Check sheet for the drawn part. Datum: minimum x, y, z corner. Units: mm. Round coordinates to 2 decimals unless told otherwise and drop trailing zeros. Write each loop counter-clockwise with the first axis right and the second up, starting at its lowest first coordinate (ties: lowest second). Pieces come first, ordered by that corner, then holes. Notation, with made-up numbers: (6.5, 12) - (64.5, 12) arc R8 cw to (64.5, 20) - close; hole circle Ø7 at (68.25, 68). An arc over 180 degrees is marked (long way). Answer as a JSON object with one key per item and string values. Group by question number.
Item 1: Sectioned sample at C-C on y = 1.1. Record the boundary of the cut face in (x, z), plus the area to 3 significant figures.
Item 2: Sectioned sample at B-B on z = 8. Record the boundary of the cut face in (x, y), plus the area to 3 significant figures.
Item 3: Sectioned sample at A-A on x = 8. Record the boundary of the cut face in (y, z).
Item 4: Release check for a two-part mould opening along Z. For the marked faces 1, 2, 3 and 4 record: pulls with the +Z half, pulls with the -Z half, needs draft (parallel to the pull), parting line crosses it, or undercut.
Item 5: Thickness scan on line 1 (X direction, y = 0.4, z = 8); line 2 (Z direction, x = 6.5, y = 1.25). Record the ranges inside material, lowest first.
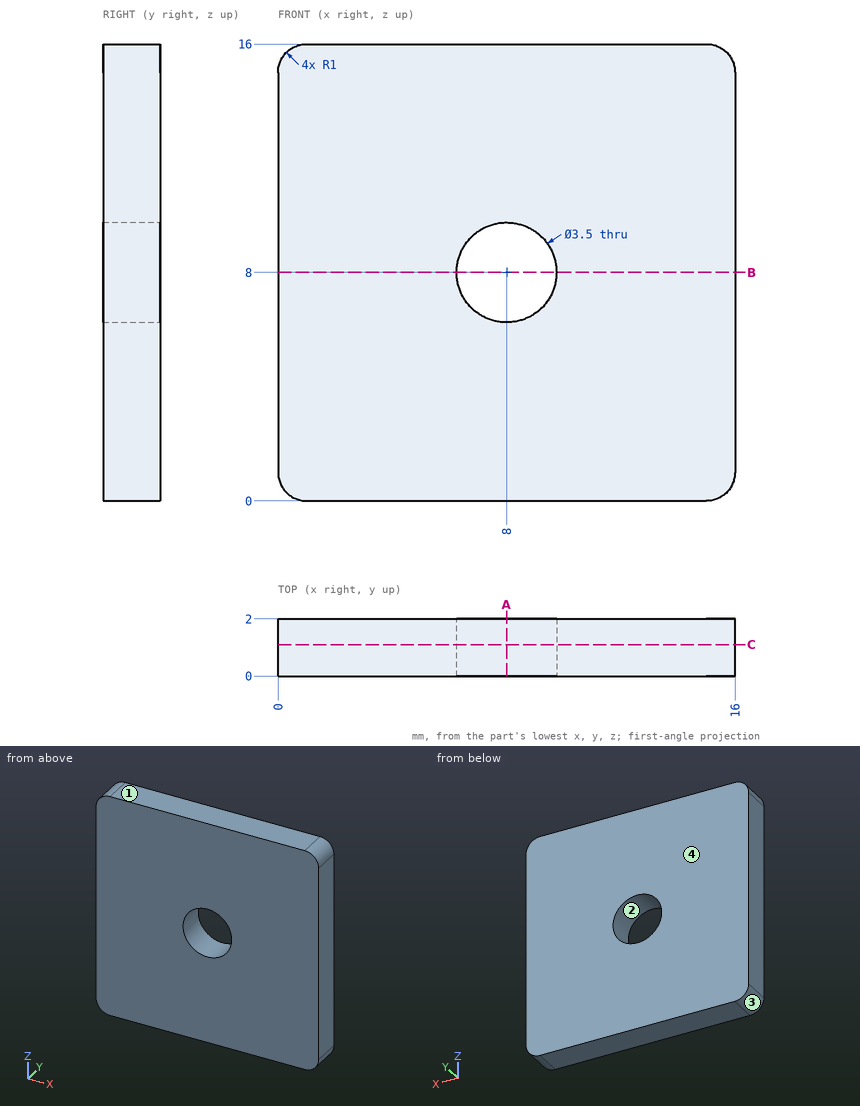
Completed:
{
 "1": {"outline": "(0, 1) arc R1 ccw to (1, 0) - (15, 0) arc R1 ccw to (16, 1) - (16, 15) arc R1 ccw to (15, 16) - (1, 16) arc R1 ccw to (0, 15) - close; hole circle Ø3.5 at (8, 8)", "area": "246 mm²"},
 "2": {"outline": "(0, 0) - (6.25, 0) - (6.25, 2) - (0, 2) - close; (9.75, 0) - (16, 0) - (16, 2) - (9.75, 2) - close", "area": "25.0 mm²"},
 "3": {"outline": "(0, 0) - (2, 0) - (2, 6.25) - (0, 6.25) - close; (0, 9.75) - (2, 9.75) - (2, 16) - (0, 16) - close"},
 "4": {"face 1": "pulls with the +Z half", "face 2": "undercut", "face 3": "pulls with the -Z half", "face 4": "needs draft"},
 "5": {"line 1": "0 to 6.25, 9.75 to 16", "line 2": "0 to 7.1, 8.9 to 16"}
}
